Geometry: final body of the model. Coordinates: model frame, mm. A direction names the side the tool comes from. Give positions to 0.01 mm unless a question says otherwise; leave off trailing zeros. Loops run counter-clockwise (first coordinate to the right, second up) from the corner with the lowest first, then second, coordinate; pieces in that order, holes last.
1. Section C-C, the plane x = -23. Output: boundary loops of the cut face in (y, z).
2. Section B-B, the plane y = -5.5. Output: boundary loops of the cut face in (x, z).
3. Section A-A, the plane y = 0. Output: boundary loops of the cut face in (x, z).
4. First-contact query: P1, Ø8, axis at x = 3, y = 1.5, coming from the -Z side; P2, Ø2, axis at y = 1.5, z = 3.5, coming from the +X side; P3, Ø4, axis at x = -16.5, y = 0.5, coming from the -Z side. Flat tips, straight axial feed; report the tip coordinate or a pass-through.
5. Draft query along Y for faces 1 (the face through (-17, 4, 5)), 2 (the face through (-25.04, 0.07, 6.65)), 3 (the face through (8, 0, 15)). Return one class per face: +Y half, -Y half, draft (parallel to the pull), parting line (faces both ways), or undercut.
6. Access query for faces 4 (the face through (-10.5, -4, 15)), 5 (the face through (-8, -0.7, 15)), 6 (the face through (-3.654, 7.014, 13.62)), 7 (the face through (-4, 2, 10)), 8 (the face through (-22, -2, 24)). Directions: +Z, -Z, +X, -X, +Y, -Y. A direction counts if a zero-diameter tool reaches every point of the face in a straight line with its end or side. Return the directions, or none.
7. Material intervals for line 1 along Z through (x, y) = (-25.4, 0); line 2 along Y through (x, z) = (-9, 15.5); line 3 along X through (y, z) = (0.5, 26.75), sorted ascending.
8. Section D-D, the plane z = 25.75. Output: boundary loops of the cut face in (x, y).
from build123d import *

# Parameters (mm, degrees)
RESSALTO_EXTRUS_O1_DEPTH   = 30
CORTE_EXTRUS_O6_DEPTH      = 17
ESBO_O6_R                  = 1.65
CORTE_EXTRUS_O4_DEPTH      = 9.7
CORTE_EXTRUS_O4_DEPTH_BACK = 8.3
CORTE_EXTRUS_O5_DEPTH      = 2
ESBO_O9_R                  = 1.65
CORTE_EXTRUS_O7_DEPTH      = 37
FILETE1_R                  = 5
ESBO_O10_R                 = 3.5
CORTE_EXTRUS_O8_DEPTH      = 22


with BuildPart() as part:
    # Esboço2 → Ressalto-extrusão1 (new body)
    with BuildSketch(Plane.XY):
        with BuildLine():
            Line((0, 8), (-28, 8))
            Line((-28, 8), (-28, -8))
            Line((-28, -8), (-10.5, -8))
            Line((-10.5, -8), (-10.5, 0.7))
            Line((-10.5, 0.7), (-4.090537862, 0.7))
            ThreePointArc((-4.090537862, 0.7), (4.15, 0), (-4.090537862, -0.7))
            Line((-4.090537862, -0.7), (-9.5, -0.7))
            Line((-9.5, -0.7), (-9.5, -8))
            Line((-9.5, -8), (0, -8))
            ThreePointArc((0, -8), (8, 0), (0, 8))
        make_face()
    extrude(amount=RESSALTO_EXTRUS_O1_DEPTH)

    # Esboço8 → Corte-extrusão6 (cut, through all)
    with BuildSketch(Plane(origin=(0, 8, 0), x_dir=(1, 0, 0), z_dir=(0, 1, 0))):
        Polygon((-22, -30), (-12, -20), (8, -20), (8, -30), align=None)
        Polygon((8, 0), (-22, 0), (-12, -10), (8, -10), align=None)
    extrude(amount=-CORTE_EXTRUS_O6_DEPTH, mode=Mode.SUBTRACT)

    # Esboço6 → Corte-extrusão4 (cut, two sides)
    with BuildSketch(Plane.XZ.offset(-0.7)) as corte_extrus_o4_sk:
        with Locations((-6.090537862, 15)):
            Circle(ESBO_O6_R)
    extrude(amount=CORTE_EXTRUS_O4_DEPTH, mode=Mode.SUBTRACT)
    extrude(corte_extrus_o4_sk.sketch, amount=-CORTE_EXTRUS_O4_DEPTH_BACK, mode=Mode.SUBTRACT)

    # Esboço7 → Corte-extrusão5 (cut)
    with BuildSketch(Plane(origin=(0, 8, 0), x_dir=(1, 0, 0), z_dir=(0, 1, 0))):
        Polygon((-2.857376354, -15), (-4.473957108, -12.2), (-7.707118616, -12.2), (-9.323699369, -15), (-7.707118616, -17.8), (-4.473957108, -17.8), align=None)
    extrude(amount=-CORTE_EXTRUS_O5_DEPTH, mode=Mode.SUBTRACT)

    # Esboço9 → Corte-extrusão7 (cut, through all)
    with BuildSketch(Plane(origin=(-28, 0, 19.455844123), x_dir=(0, 0, -1), z_dir=(1, 0, 0))):
        with Locations((14.455844123, 0)):
            Circle(ESBO_O9_R)
        with Locations((-5.544155877, 0)):
            Circle(ESBO_O9_R)
    extrude(amount=CORTE_EXTRUS_O7_DEPTH, mode=Mode.SUBTRACT)

    # Filete1
    filete1_edges = [part.edges().sort_by_distance(p)[0] for p in [
        (-25, -8, 0),
        (-25, 8, 30),
        (-25, -8, 30),
        (-25, 8, 0),
    ]]
    fillet(filete1_edges, radius=FILETE1_R)

    # Esboço10 → Corte-extrusão8 (cut)
    with BuildSketch(Plane(origin=(0, 0, 0), x_dir=(0, 0, -1), z_dir=(1, 0, 0))):
        with Locations((-25, 0)):
            Circle(ESBO_O10_R)
        with Locations((-5, 0)):
            Circle(ESBO_O10_R)
    extrude(amount=-CORTE_EXTRUS_O8_DEPTH, mode=Mode.SUBTRACT)


solid = part.part
Answers below:
1. outline: (-8, 5) arc R5 ccw to (-3, 0) - (3, 0) arc R5 ccw to (8, 5) - (8, 25) arc R5 ccw to (3, 30) - (-3, 30) arc R5 ccw to (-8, 25) - close; hole circle Ø3.3 at (0, 5); hole circle Ø3.3 at (0, 25)
2. outline: (-28, 0.67) - (-21.33, 0.67) - (-12, 10) - (-10.5, 10) - (-10.5, 20) - (-12, 20) - (-21.33, 29.33) - (-28, 29.33) - close; (-9.5, 10) - (5.81, 10) - (5.81, 20) - (-9.5, 20) - close; hole circle Ø3.3 at (-6.09, 15)
3. outline: (-28, 0) - (-22, 0) - (-20.5, 1.5) - (-22, 1.5) - (-22, 3.35) - (-28, 3.35) - close; (-28, 6.65) - (-22, 6.65) - (-22, 8.5) - (-13.5, 8.5) - (-12, 10) - (-10.5, 10) - (-10.5, 20) - (-12, 20) - (-13.5, 21.5) - (-22, 21.5) - (-22, 23.35) - (-28, 23.35) - close; (-28, 26.65) - (-22, 26.65) - (-22, 28.5) - (-20.5, 28.5) - (-22, 30) - (-28, 30) - close; (4.15, 10) - (8, 10) - (8, 20) - (4.15, 20) - close
4. P1: stops at z = 10
4. P2: stops at x = -22
4. P3: stops at z = 7.45
5. face 1: draft
5. face 2: undercut
5. face 3: parting line
6. face 4: +Z, -Z, -Y
6. face 5: +Z, -Z
6. face 6: +Y
6. face 7: -Z, +X, +Y, -Y
6. face 8: +X
7. line 1: z = 0 to 3.35, 6.65 to 23.35, 26.65 to 30
7. line 2: y = -8 to -0.7, 0.7 to 6
7. line 3: x = -28 to -22
8. outline: (-28, -7.94) - (-17.75, -7.94) - (-17.75, -3.42) - (-22, -3.42) - (-22, -1.47) - (-28, -1.47) - close; (-28, 1.47) - (-22, 1.47) - (-22, 3.42) - (-17.75, 3.42) - (-17.75, 7.94) - (-28, 7.94) - close
